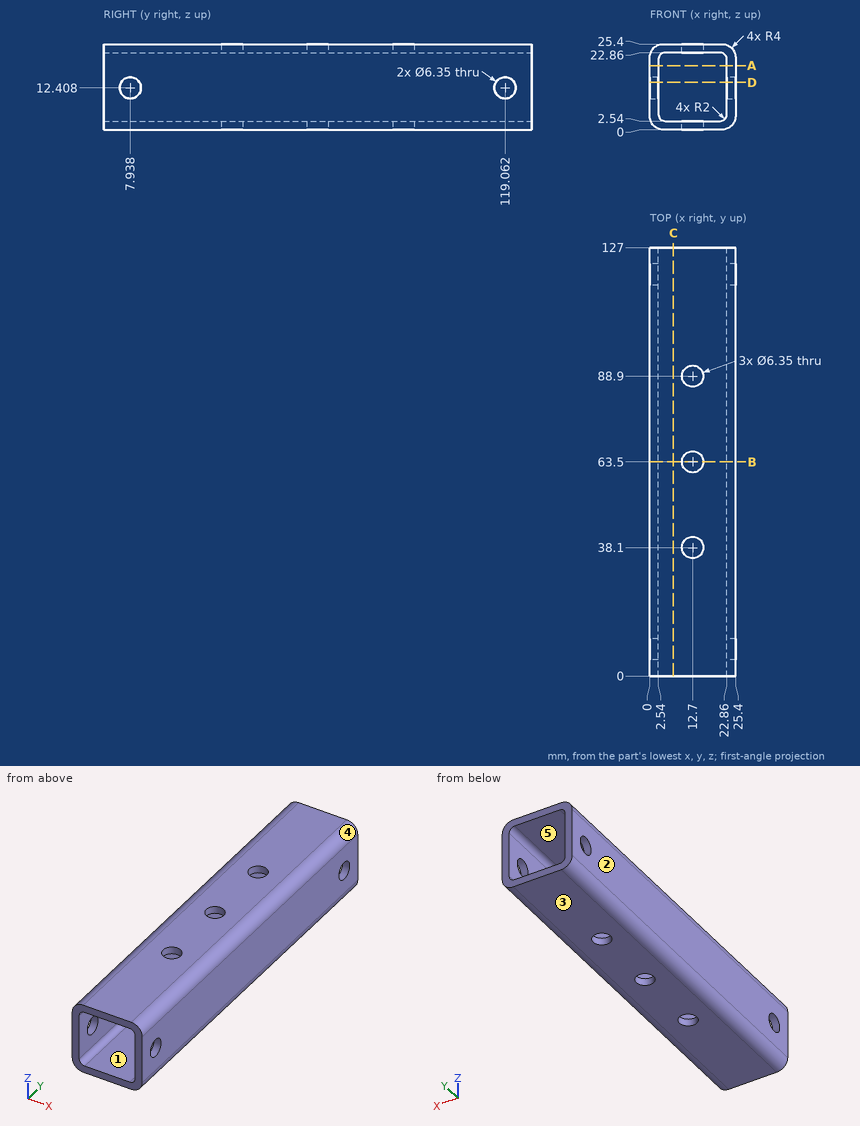
Could you check a few things on this drawing? It's one solid part, dimensions in mm from its lowest x, y, z. A direction names the side the tool comes from. Give positions to 0.01 mm unless a question says otherwise; leave off trailing zeros. Write each loop counter-clockwise with the first axis right and the second up, starting at its lowest first coordinate (ties: lowest second). Pieces come first, ordered by that corner, then holes. Notation, with made-up numbers: M 76.5,70 L 113.5,70 A21 cw 113.5,106 Z; hole C 41.5,54.25 d4. An arc over 180 degrees is marked long. Put each result on its own line as item: value. Start each with the question number.
Item 1: Thinking about a two-plate mould opening in X: for the marked faces 3, 4 and 5, which applies, +X half, -X half, draft (parallel to the pull), parting line (faces both ways), or undercut?
Item 2: If we section it at A-A, the plane z = 19: Write out the boundary of the cut face in (x, y).
Item 3: If we section it at B-B, the plane y = 63.5: Write out the boundary of the cut face in (x, z) (1 decimal), then the cut area to 3 significant figures.
Item 4: If we section it at C-C, the plane x = 7: Write out the boundary of the cut face in (y, z).
Item 5: If we section it at D-D, the plane z = 14: Write out the boundary of the cut face in (x, y) (1 decimal).
Item 6: On a 3-axis mill with a long thin cutter (end or side, diameter ignored), from which of +Z, -Z, +X, -X, +Y, -Y can I reach the whole of each face in a straight line? I mean the marked faces 1 and 2. Say none if no direction works.
Item 7: I need wall thicknesses on L1, parallel to X at y = 87.5, z = 21 (1 decimal); L2, parallel to Z at x = 13.25, y = 22; L3, parallel to Z at x = 4.25, y = 87.5. Which ranges of each line are inside material? Lowest first, please. Write a range as from..to.
Item 8: Will this pin go through, and if not, where does the flat tip stop? pin 1 (10 mm diameter, centred on x = 12.7, y = 63.5, fed in from +Z).
Values:
1. face 3: draft
1. face 4: +X half
1. face 5: undercut
2. outline: M 0,0 L 2.54,0 L 2.54,127 L 0,127 Z; M 22.86,0 L 25.4,0 L 25.4,127 L 22.86,127 Z
3. outline: M 0,4 A4 ccw 4,0 L 9.5,0 L 9.5,2.5 L 4.5,2.5 A2 cw 2.5,4.5 L 2.5,20.9 A2 cw 4.5,22.9 L 9.5,22.9 L 9.5,25.4 L 4,25.4 A4 ccw 0,21.4 Z; M 15.9,0 L 21.4,0 A4 ccw 25.4,4 L 25.4,21.4 A4 ccw 21.4,25.4 L 15.9,25.4 L 15.9,22.9 L 20.9,22.9 A2 cw 22.9,20.9 L 22.9,4.5 A2 cw 20.9,2.5 L 15.9,2.5 Z
3. area: 190 mm²
4. outline: M 0,0 L 127,0 L 127,2.54 L 0,2.54 Z; M 0,22.86 L 127,22.86 L 127,25.4 L 0,25.4 Z
5. outline: M 0,0 L 2.5,0 L 2.5,5.2 L 0,5.2 Z; M 0,10.7 L 2.5,10.7 L 2.5,116.3 L 0,116.3 Z; M 0,121.8 L 2.5,121.8 L 2.5,127 L 0,127 Z; M 22.9,0 L 25.4,0 L 25.4,5.2 L 22.9,5.2 Z; M 22.9,10.7 L 25.4,10.7 L 25.4,116.3 L 22.9,116.3 Z; M 22.9,121.8 L 25.4,121.8 L 25.4,127 L 22.9,127 Z
6. face 1: +Y, -Y
6. face 2: +Z, -Z, -X, +Y, -Y
7. L1: 0..2.5, 22.9..25.4
7. L2: 0..2.54, 22.86..25.4
7. L3: 0..2.56, 22.84..25.4
8. pin 1: z = 25.4
